Part model, mm, in its own coordinate system. Give positions to 0.01 mm unless a question says otherwise; leave off trailing zeros. Order: outer loops, then holes, each group sorted by start corner. A loop starts at its lowest first (then second) coordinate and runs counter-clockwise, first axis right, second up. Notation, with made-up numbers: M 81.25,65.25 L 134.25,65.25 A11 ccw 134.25,71.25 Z; hole C 17,48 d11. An arc over 180 degrees is marked long. Answer as a JSON object with one key per item and string values.
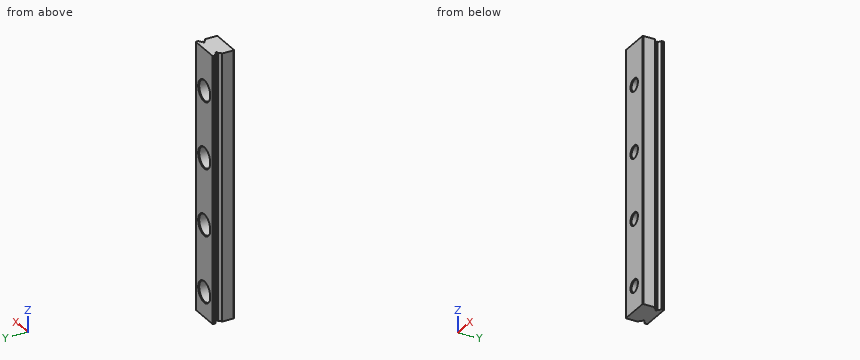
from build123d import *

# Parameters (mm, degrees)
EXTRUDE1_DEPTH                     = 80
HOLE_WIZARD_M3_1_D                 = 3.5
HOLE_WIZARD_M3_1_CBORE_D           = 6
HOLE_WIZARD_M3_1_CBORE_DEPTH       = 4.5
CHAMFER_1_SIZE                     = 0.2
PATTERN_LINEAR_1_COUNT             = 4
PATTERN_LINEAR_1_PITCH             = 20
CHAMFER_1_OF_PATTERN_LINEAR_1_SIZE = 0.2


with BuildPart() as part:
    # Sketch1 → Extrude1 (new body)
    with BuildSketch(Plane.XY):
        with BuildLine():
            Line((-4.3, -3.25), (4.3, -3.25))
            Line((4.3, -3.25), (4.5, -3.05))
            Line((4.5, -3.05), (4.5, 0.455012563))
            ThreePointArc((4.5, 0.455012563), (3.948817336, 0.691078965), (3.631754163, 1.2))
            Line((3.631754163, 1.2), (3.131754163, 1.2))
            Line((3.131754163, 1.2), (3.131754163, 1.7))
            Line((3.131754163, 1.7), (3.631754163, 1.7))
            ThreePointArc((3.631754163, 1.7), (3.948817336, 2.208921035), (4.5, 2.444987437))
            Line((4.5, 2.444987437), (4.5, 3.05))
            Line((4.5, 3.05), (4.3, 3.25))
            Line((4.3, 3.25), (-4.3, 3.25))
            Line((-4.3, 3.25), (-4.5, 3.05))
            Line((-4.5, 3.05), (-4.5, 2.444987437))
            ThreePointArc((-4.5, 2.444987437), (-3.948817336, 2.208921035), (-3.631754163, 1.7))
            Line((-3.631754163, 1.7), (-3.131754163, 1.7))
            Line((-3.131754163, 1.7), (-3.131754163, 1.2))
            Line((-3.131754163, 1.2), (-3.631754163, 1.2))
            ThreePointArc((-3.631754163, 1.2), (-3.948817336, 0.691078965), (-4.5, 0.455012563))
            Line((-4.5, 0.455012563), (-4.5, -3.05))
            Line((-4.5, -3.05), (-4.3, -3.25))
        make_face()
    extrude(amount=EXTRUDE1_DEPTH)

    # M3 平盤頭機械螺釘的柱孔1 (through all)
    with Locations(Plane(origin=(0, 3.25, 0), x_dir=(1, 0, 0), z_dir=(0, 1, 0))):
        with Locations((0, -7.5)):
            hole_wizard_m3_1 = CounterBoreHole(HOLE_WIZARD_M3_1_D / 2, HOLE_WIZARD_M3_1_CBORE_D / 2, HOLE_WIZARD_M3_1_CBORE_DEPTH)

    # 導角1
    chamfer_1_edges = [part.edges().sort_by_distance(p)[0] for p in [
        (-3, 3.25, 7.5),
        (1.75, -3.25, 7.5),
    ]]
    chamfer(chamfer_1_edges, length=CHAMFER_1_SIZE)

    # 直線複製排列1: M3 平盤頭機械螺釘的柱孔1 ×4
    with Locations(*[(0, 0, i * PATTERN_LINEAR_1_PITCH) for i in range(1, PATTERN_LINEAR_1_COUNT)]):
        add(hole_wizard_m3_1, mode=Mode.SUBTRACT)

    # 導角1 of 直線複製排列1
    chamfer_1_of_pattern_linear_1_edges = [part.edges().sort_by_distance(p)[0] for p in [
        (-3, 3.25, 27.5),
        (1.75, -3.25, 27.5),
        (-3, 3.25, 47.5),
        (1.75, -3.25, 47.5),
        (-3, 3.25, 67.5),
        (1.75, -3.25, 67.5),
    ]]
    chamfer(chamfer_1_of_pattern_linear_1_edges, length=CHAMFER_1_OF_PATTERN_LINEAR_1_SIZE)


solid = part.part
1. Cut at C-C on x = 0. State how many separate pieces and enclosed holes the cut face has, plus the area to 3 significant figures.
Worked answers:
{"separate pieces": "5", "enclosed holes": "0", "area": "384 mm^2"}
2. Pin check, flat tips, straight feed: P1, Ø1.8, axis at x = 0.5, z = 6.5, coming from the +Y side; P2, Ø5, axis at x = 0, z = 47.5, coming from the -Y side. Stop position of each tip, or through.
Worked answers:
{"P1": "stops at y = -1.25", "P2": "stops at y = -3.25"}
3. Cut at B-B on z = 16. Give the cut face in (x, y), plus the area to 3 significant figures.
Worked answers:
{"outline": "M -4.5,-3.05 L -4.3,-3.25 L 4.3,-3.25 L 4.5,-3.05 L 4.5,0.46 A1 cw 3.63,1.2 L 3.13,1.2 L 3.13,1.7 L 3.63,1.7 A1 cw 4.5,2.44 L 4.5,3.05 L 4.3,3.25 L -4.3,3.25 L -4.5,3.05 L -4.5,2.44 A1 cw -3.63,1.7 L -3.13,1.7 L -3.13,1.2 L -3.63,1.2 A1 cw -4.5,0.46 Z", "area": "55.2 mm^2"}
4. Probe line 1 along Z through (x, y) = (0, 0.2); line 2 along Z through (x, y) = (0, -1.7); line 3 along X through (y, z) = (-1.6, 7.5). List the from-to ranges inside material, lowest first.
Worked answers:
{"line 1": "z = 0 to 4.5, 10.5 to 24.5, 30.5 to 44.5, 50.5 to 64.5, 70.5 to 80", "line 2": "z = 0 to 5.75, 9.25 to 25.75, 29.25 to 45.75, 49.25 to 65.75, 69.25 to 80", "line 3": "x = -4.5 to -1.75, 1.75 to 4.5"}
